Can you work these out from the model? Positions are in its coordinate system, mm. Coordinates: 2 decimals unless noted, no trailing zeros. Loops run counter-clockwise (first coordinate to the right, second up) from the corner with the lowest first, then second, coordinate; pieces in that order, holes last.
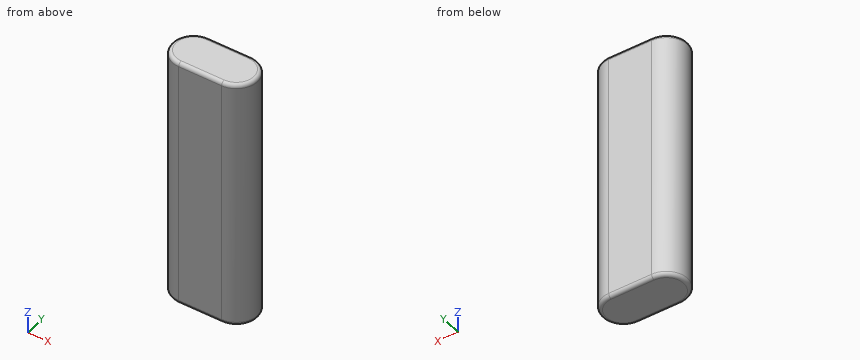
Autodesk Inventor part; units mm, degrees
ref_plane "YZ Plane" through (0, 0, 0) normal (1, 0, 0) x (0, 1, 0)
ref_plane "XZ Plane" through (0, 0, 0) normal (0, 1, 0) x (-1, 0, 0)
ref_plane "XY Plane" through (0, 0, 0) normal (0, 0, 1) x (1, 0, 0)
sketch "スケッチ1" plane through (0, 0, 0) normal (0, 0, 1) x (1, 0, 0)
  line L0 (-11.8937, 2.2764) -> (11.4063, 2.2764) construction
  line L1 (-11.8937, 13.6264) -> (11.4063, 13.6264)
  line L2 (11.4063, -9.0736) -> (-11.8937, -9.0736)
  arc A0 (-11.8937, 13.6264) -> (-11.8937, -9.0736) centre (-11.8937, 2.2764) ccw
  arc A1 (11.4063, -9.0736) -> (11.4063, 13.6264) centre (11.4063, 2.2764) ccw
  point P0 (0, 0)
  point P1 (-0.2437, 2.2764)
  dimension "d0" = 46
  dimension "d1" = 22.7
extrude "押し出し1" add sketch "スケッチ1" along normal blind 136.7
fillet "フィレット1" radius 2 8 edges at (-0.2437, 13.6264, 136.7) (-23.2437, 2.2764, 136.7) (-0.2437, -9.0736, 136.7) (22.7563, 2.2764, 136.7) (-0.2437, -9.0736, 0) (-23.2437, 2.2764, 0) (-0.2437, 13.6264, 0) (22.7563, 2.2764, 0)
properties part number "バッテリー"
Item 1: I'm going to push flat-ended pins straight in: P1, Ø3, axis at y = 11, z = 38.5, coming from the -X side; P2, Ø1.5, axis at y = 3.5, z = 96, coming from the -X side; P3, Ø10, axis at y = 0.5, z = 91, coming from the +X side; P4, Ø6, axis at y = -4.5, z = 77.5, coming from the -X side. Where does each tip first touch, or does it pass through?
Results are:
P1: stops at x = -20.65
P2: stops at x = -23.23
P3: stops at x = 22.76
P4: stops at x = -22.6
Item 2: I need wall thicknesses on line 1 along Y through (x, z) = (12, 116); line 2 along Z through (x, y) = (21, 2.75); line 3 along Y through (x, z) = (-17, 24.5). Which ranges of each line are inside material? Lowest first, please.
Results are:
line 1: y = -9.06 to 13.61
line 2: z = 0.02 to 136.68
line 3: y = -7.86 to 12.41
Item 3: Suppose I cut it at A-A, the plane z = 85. Please give me the cut outline in (x, y).
Results are:
outline: (-11.89, -9.07) - (11.41, -9.07) arc R11.35 ccw to (11.41, 13.63) - (-11.89, 13.63) arc R11.35 ccw to start
